Could you check a few things on this model? Use its own coordinates, in mm. Face numbers are marked on the shaded views. Give positions to 0.01 mm unless a question says otherwise; leave off trailing zeros. Order: outer loops, then holes, each group sorted by start corner. A loop starts at its lowest first (then second) coordinate and runs counter-clockwise, first axis right, second up. Notation, with made-up numbers: M -40,27 L -24,27 A12 ccw -24,37 Z; hole C -12,30.25 d9. An arc over 180 degrees is marked long. Use a Markdown table: item, result. Add a question column.
Item 1: Suppose I cut it at D-D on z = 19. Write out the boundary of the cut face in (x, y), plus the area to 3 significant figures.
Item 2: Suppose I cut it at B-B on x = -13.75. Write out the boundary of the cut face in (y, z).
Item 3: If we mould it in two halves opening along Y, with no side actions, what happens to the marked faces 1, 2, 3 and 4? For each: released by +Y, released by -Y, zero draft, split by the parting line, or undercut.
Item 4: I'm going to push flat-ended pins straight in: pin 1 Ø2.5 at (y, z) = (-5, 22) entering from +X; pin 2 Ø0.5 at (y, z) = (-5, 10.5) entering from +X; pin 3 Ø2 at (y, z) = (-6, 11.5) entering from +X. Where does each tip first touch, or does it pass through?
Item 5: If I drill on L1, parallel to Z at x = -13.5, y = -6.5; L2, parallel to Z at x = -10.75, y = -4.5; L3, parallel to Y at x = -13.75, z = 18.25, over which ranges is the centre line in solid material (lowest first)? Write a range as from..to.
Item 6: Suppose I cut it at A-A on z = 23.25. Write out the boundary of the cut face in (x, y), plus the area to 3 significant figures.
Item 7: Suppose I cut it at C-C on x = -6. Write out the boundary of the cut face in (y, z), plus the area to 3 significant figures.
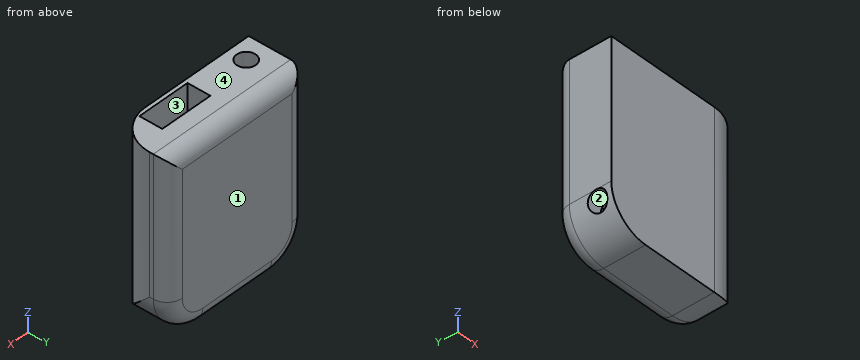
from build123d import *

# Parameters (mm, degrees)
F0_W         = 20
F0_H         = 23
F1_DEPTH     = 7
F2_W         = 15
F2_H         = 3
F3_DEPTH     = 3
F4_W         = 7
F4_H         = 17
F5_DEPTH     = 3
F6_W         = 3
F6_H         = 1
F7_DEPTH     = 3
F8_W         = 2.5268201925
F8_H         = 2
F9_DEPTH     = 3
F10_R        = 1.25
F11_DEPTH    = 5
F12_R        = 2
F13_W        = 5.6845681682
F13_H        = 12.7295220874
F14_DEPTH    = 3
F15_W        = 20
F15_H        = 23
F16_DEPTH    = 0.5
F17_T1_DEPTH = 20
F17_T3_DEPTH = 48
F17_T6_ANGLE = 90
F17_T8_ANGLE = 90
F18_R        = 1.25
F19_DEPTH    = 7


# Not quite as in the source:
# - a fillet or chamfer that OpenCascade refuses, or shapes differently, is made with other operations: its cross-section is extruded or revolved along the edge and cut away or added


with BuildPart() as f1:
    # F0 (on Front) → F1 (new body)
    with BuildSketch(Plane.XZ):
        with Locations((-9.5134219155, 16.3173061975)):
            Rectangle(F0_W, F0_H)
    extrude(amount=F1_DEPTH)

    # F2 (on face) → F3 (cut)
    with BuildSketch(Plane.XZ.offset(7)):
        with Locations((-10.0134219155, 8.3173061975)):
            Rectangle(F2_W, F2_H)
    extrude(amount=-F3_DEPTH, mode=Mode.SUBTRACT)

    # F4 (on face) → F5 (cut)
    with BuildSketch(Plane.XZ.offset(7)):
        with Locations((-6.5459148027, 19.3173061975)):
            Rectangle(F4_W, F4_H)
    extrude(amount=-F5_DEPTH, mode=Mode.SUBTRACT)

    # F6 (on face) → F7 (cut)
    with BuildSketch(Plane.XZ.offset(7)):
        with Locations((-6.5459148027, 10.3173061975)):
            Rectangle(F6_W, F6_H)
    extrude(amount=-F7_DEPTH, mode=Mode.SUBTRACT)

    # F8 (on face) → F9 (cut)
    with BuildSketch(Plane.XZ.offset(7)):
        with Locations((-11.3093248989, 13.8173061975)):
            Rectangle(F8_W, F8_H)
    extrude(amount=-F9_DEPTH, mode=Mode.SUBTRACT)

    # F10 (on face) → F11 (cut)
    with BuildSketch(Plane(origin=(-19.5134219155, 0, 0), x_dir=(0, -1, 0), z_dir=(-1, 0, 0))):
        with Locations((5.55, 8.5673061975)):
            Circle(F10_R)
    extrude(amount=-F11_DEPTH, mode=Mode.SUBTRACT)

    # F12
    f12_edges = [f1.edges().sort_by_distance(p)[0] for p in [
        (0.486578, 0, 16.317306),
        (-19.513422, 0, 16.317306),
        (-9.513422, 0, 27.817306),
        (-9.513422, 0, 4.817306),
    ]]
    fillet(f12_edges, radius=F12_R)

    # F13 (on face) → F14 (cut)
    with BuildSketch(Plane.XZ.offset(7)):
        with Locations((-15.4150190793, 19.1820672412)):
            Rectangle(F13_W, F13_H)
    extrude(amount=-F14_DEPTH, mode=Mode.SUBTRACT)

    # F15 (on face) → F16 (join)
    with BuildSketch(Plane.XZ.offset(7)):
        with Locations((-9.5134219155, 16.3173061975)):
            Rectangle(F15_W, F15_H)
    extrude(amount=F16_DEPTH)

    # F17: fillet of radius 5 on 3 edges, made by hand

    # F17_s2 → F17_t1 (cut)
    with BuildSketch(Plane.XZ):
        with BuildLine():
            ThreePointArc((-19.5134219155, 9.8173061975), (-18.0489558214, 6.2817722916), (-14.5134219155, 4.8173061975))
            Line((-14.5134219155, 4.8173061975), (-19.5134219155, 4.8173061975))
            Line((-19.5134219155, 4.8173061975), (-19.5134219155, 9.8173061975))
        make_face()
        with BuildLine():
            ThreePointArc((0.4865780845, 9.8173061975), (-0.9778880095, 6.2817722916), (-4.5134219155, 4.8173061975))
            Line((-4.5134219155, 4.8173061975), (0.4865780845, 4.8173061975))
            Line((0.4865780845, 4.8173061975), (0.4865780845, 9.8173061975))
        make_face()
    extrude(amount=F17_T1_DEPTH, mode=Mode.SUBTRACT)

    # F17_s4 → F17_t3 (cut)
    with BuildSketch(Plane.XY.offset(-7.6826938025)):
        with BuildLine():
            ThreePointArc((0.4865780845, -2.5), (-0.9778880095, -6.0355339059), (-4.5134219155, -7.5))
            Line((-4.5134219155, -7.5), (0.4865780845, -7.5))
            Line((0.4865780845, -7.5), (0.4865780845, -2.5))
        make_face()
    extrude(amount=F17_T3_DEPTH, mode=Mode.SUBTRACT)

    # F17_s5 → F17_t6 (revolve, cut)
    with BuildSketch(Plane.XY.offset(9.8173061975)):
        with BuildLine():
            ThreePointArc((-1.5134219155, 0), (-0.0992083531, -0.5857864376), (0.4865780845, -2))
            Line((0.4865780845, -2), (0.4865780845, 0))
            Line((0.4865780845, 0), (-1.5134219155, 0))
        make_face()
    revolve(axis=Axis((-4.5134219155, 0, 9.8173061975), (0, 1, 0)), revolution_arc=F17_T6_ANGLE, mode=Mode.SUBTRACT)

    # F17_s7 → F17_t8 (revolve, cut)
    with BuildSketch(Plane.YZ.offset(-14.5134219155)):
        with BuildLine():
            ThreePointArc((0, 6.8173061975), (-0.5857864376, 5.4030926351), (-2, 4.8173061975))
            Line((-2, 4.8173061975), (0, 4.8173061975))
            Line((0, 4.8173061975), (0, 6.8173061975))
        make_face()
    revolve(axis=Axis((-14.5134219155, 0, 9.8173061975), (0, 1, 0)), revolution_arc=F17_T8_ANGLE, mode=Mode.SUBTRACT)

    # F18 (on face) → F19 (cut)
    with BuildSketch(Plane.XY.offset(27.8173061975)):
        with Locations((-16.5796671063, -5.1869219169)):
            Circle(F18_R)
    extrude(amount=-F19_DEPTH, mode=Mode.SUBTRACT)


solid = f1.part
Findings below:
| question | item | result |
|---|---|---|
| 1 | outline | M -19.51,-7.5 L -4.51,-7.5 A5 ccw 0.49,-2.5 L 0.49,-2 A2 ccw -1.51,0 L -17.51,0 A2 ccw -19.51,-2 Z; hole M -18.26,-7 L -12.57,-7 L -12.57,-4 L -18.26,-4 Z; hole M -10.05,-7 L -3.05,-7 L -3.05,-4 L -10.05,-4 Z |
| 1 | area | 105 mm^2 |
| 2 | outline | M -7.5,4.82 L -2,4.82 A2 ccw 0,6.82 L 0,25.82 A2 ccw -2,27.82 L -7.5,27.82 Z; hole M -7,6.82 L -4,6.82 L -4,9.82 L -7,9.82 Z; hole M -7,12.82 L -4,12.82 L -4,25.55 L -7,25.55 Z |
| 3 | face 1 | released by +Y |
| 3 | face 2 | undercut |
| 3 | face 3 | undercut |
| 3 | face 4 | zero draft |
| 4 | pin 1 | stops at x = 0.33 |
| 4 | pin 2 | stops at x = -0.05 |
| 4 | pin 3 | stops at x = -0.18 |
| 5 | L1 | z = 4.82..6.82, 9.82..12.82, 25.55..27.82 |
| 5 | L2 | z = 4.82..6.82, 9.82..12.82, 14.82..27.82 |
| 5 | L3 | y = -7.5..-7, -4..0 |
| 6 | outline | M -19.51,-7.5 L -4.51,-7.5 A5 ccw 0.49,-2.5 L 0.49,-2 A2 ccw -1.51,0 L -17.51,0 A2 ccw -19.51,-2 Z; hole M -18.26,-7 L -12.57,-7 L -12.57,-4 L -16.19,-4 A1.25 ccw -16.97,-4 L -18.26,-4 Z; hole M -10.05,-7 L -3.05,-7 L -3.05,-4 L -10.05,-4 Z |
| 6 | area | 105 mm^2 |
| 7 | outline | M -7.5,4.82 L -2,4.82 A2 ccw 0,6.82 L 0,25.82 A2 ccw -2,27.82 L -4,27.82 L -4,6.82 L -7,6.82 L -7,27.82 L -7.5,27.82 Z |
| 7 | area | 108 mm^2 |
